Design review of the part built by this model. Coordinates are the model's own, in mm. Give positions to 0.01 mm unless a question says otherwise; leave off trailing zeros. Loops run counter-clockwise (first coordinate to the right, second up) from the corner with the lowest first, then second, coordinate; pieces in that order, holes last. Notation, with made-up numbers: (28.25, -27.75) -> (47.25, -27.75) arc R36 ccw to (47.25, 8.25) -> close; hole circle Ø11 at (-36.75, 40.5). An arc over 180 degrees is marked (long way). Answer in a Markdown table with one row per item. Add a question column.
(1) For line 1 (Y direction, x = -121.9, z = -0.15); line 2 (Y direction, x = -121.9, z = 0.45); line 3 (Y direction, x = -125, z = -2), list the stretches that pass through material, from the lowest coordinate up.
(2) Consider section B-B on z = -4.5. Write out the cut boundary in (x, y).
(3) Consider section A-A on x = 53.5. Write out the cut boundary in (y, z).
(4) For pin 1 (1.2 mm diameter, centred on y = 10.5, z = -1.5, fed in from +X); pin 2 (5 mm diameter, centred on x = -85.5, y = 19, fed in from -Z); pin 3 (2 mm diameter, centred on x = 99.5, y = 19, fed in from +Z); pin 4 (1 mm diameter, centred on x = 165.5, z = 0.5, fed in from +Y), all flat-tipped, find the tip position at first contact; note any pin that passes through.
from build123d import *

# Parameters (mm, degrees)
BOSS_EXTRUDE1_START        = 8
SKETCH2_W                  = 381
SKETCH2_H                  = 2
BOSS_EXTRUDE1_DEPTH        = 37
SKETCH3_W                  = 345
SKETCH3_H                  = 2
BOSS_EXTRUDE2_DEPTH        = 6
SKETCH4_W                  = 40.623
SKETCH4_H                  = 17.5
CUT_EXTRUDE1_DEPTH         = 3
F_6_CLEARANCE_HOLE1_D      = 3.6576
FILLET2_R                  = 5
FILLET3_R                  = 3
SKETCH8_W                  = 2
SKETCH8_H                  = 4
CUT_EXTRUDE2_DEPTH         = 196.834751768
FLATTEN_BENDS1_START       = -7
FLATTEN_BENDS1_OUTLINE_W   = 345
FLATTEN_BENDS1_OUTLINE_H   = 2
FLATTEN_BENDS1_DEPTH       = 6
FLATTEN_BENDS1_START_2     = -1
FLATTEN_BENDS1_2_OUTLINE_W = 345
FLATTEN_BENDS1_2_OUTLINE_H = 4.701769682
FLATTEN_BENDS1_2_DEPTH     = 2
PROCESS_BENDS1_START       = -172.5
PROCESS_BENDS1_DEPTH       = 345
PROCESS_BENDS1_2_DEPTH     = 345


# Read off the part's stored shape, not the designer's step: Flatten-Bends1, Process-Bends1
with BuildPart() as part:
    # Sketch2 → Boss-Extrude1 (new body)
    with BuildSketch(Plane(origin=(0, 0, 0), x_dir=(1, 0, 0), z_dir=(0, 1, 0)).offset(BOSS_EXTRUDE1_START)):
        Rectangle(SKETCH2_W, SKETCH2_H)
    extrude(amount=BOSS_EXTRUDE1_DEPTH)

    # Sketch3 → Boss-Extrude2 (add)
    with BuildSketch(Plane(origin=(0, 0, -1), x_dir=(-1, 0, 0), z_dir=(0, 0, -1))):
        with Locations((0, 9)):
            Rectangle(SKETCH3_W, SKETCH3_H)
    extrude(amount=BOSS_EXTRUDE2_DEPTH)

    # Sketch4 → Cut-Extrude1 (cut)
    with BuildSketch(Plane.XY.offset(1)):
        with Locations((170.1885, 36.25)):
            Rectangle(SKETCH4_W, SKETCH4_H)
        with Locations((-170.1885, 36.25)):
            Rectangle(SKETCH4_W, SKETCH4_H)
    extrude(amount=-CUT_EXTRUDE1_DEPTH, mode=Mode.SUBTRACT)

    # #6 Clearance Hole1 (through all)
    with Locations(Plane.XY.offset(1)):
        with Locations((-121.9, 35), (-121.9, 19), (-85.5, 35), (-85.5, 19), (99.5, 19), (99.5, 35), (135.9, 35), (135.9, 19)):
            Hole(F_6_CLEARANCE_HOLE1_D / 2)

    # Fillet2
    fillet2_edges = [part.edges().sort_by_distance(p)[0] for p in [
        (-190.5, 27.5, 0),
        (-149.877, 45, 0),
        (190.5, 27.5, 0),
        (149.877, 45, 0),
        (-190.5, 8, 0),
        (190.5, 8, 0),
    ]]
    fillet(fillet2_edges, radius=FILLET2_R)

    # Fillet3
    fillet3_edges = [part.edges().sort_by_distance(p)[0] for p in [
        (-149.877, 27.5, 0),
        (149.877, 27.5, 0),
    ]]
    fillet(fillet3_edges, radius=FILLET3_R)

    # Sketch8 → Cut-Extrude2 (cut, through all)
    with BuildSketch(Plane(origin=(0, 0, -1), x_dir=(-1, 0, 0), z_dir=(0, 0, -1))):
        with Locations((173.5, 10)):
            Rectangle(SKETCH8_W, SKETCH8_H)
        with Locations((-173.5, 10)):
            Rectangle(SKETCH8_W, SKETCH8_H)
    extrude(amount=-CUT_EXTRUDE2_DEPTH, mode=Mode.SUBTRACT)

    # Flatten-Bends1 outline → Flatten-Bends1 (cut)
    with BuildSketch(Plane.XY.offset(FLATTEN_BENDS1_START)):
        with Locations((0, 9)):
            Rectangle(FLATTEN_BENDS1_OUTLINE_W, FLATTEN_BENDS1_OUTLINE_H)
    extrude(amount=FLATTEN_BENDS1_DEPTH, mode=Mode.SUBTRACT)

    # Flatten-Bends1 2 outline → Flatten-Bends1 2 (add)
    with BuildSketch(Plane.XY.offset(FLATTEN_BENDS1_START_2)):
        with Locations((0, 5.649115159)):
            Rectangle(FLATTEN_BENDS1_2_OUTLINE_W, FLATTEN_BENDS1_2_OUTLINE_H)
    extrude(amount=FLATTEN_BENDS1_2_DEPTH)

    # Process-Bends1 outline → Process-Bends1 (cut)
    with BuildSketch(Plane.YZ.offset(PROCESS_BENDS1_START)):
        with BuildLine():
            Line((3.298230318, -1), (8.171572875, -1))
            ThreePointArc((8.171572875, -1), (9.267949192, 0.449489743), (11, 1))
            Line((11, 1), (3.298230318, 1))
            Line((3.298230318, 1), (3.298230318, -1))
        make_face()
    extrude(amount=PROCESS_BENDS1_DEPTH, mode=Mode.SUBTRACT)

    # Process-Bends1 2 outline → Process-Bends1 2 (add)
    with BuildSketch(Plane.YZ.offset(PROCESS_BENDS1_START)):
        with BuildLine():
            Line((8, -2), (8, -7))
            Line((8, -7), (10, -7))
            Line((10, -7), (10, -2))
            ThreePointArc((10, -2), (10.292893219, -1.292893219), (11, -1))
            Line((11, -1), (8.171572875, -1))
            ThreePointArc((8.171572875, -1), (8.043204321, -1.492694064), (8, -2))
        make_face()
    extrude(amount=PROCESS_BENDS1_2_DEPTH)


solid = part.part
Values follow:
| question | item | result |
|---|---|---|
| 1 | line 1 | 8.64 to 17.17, 20.83 to 33.17, 36.83 to 45 |
| 1 | line 2 | 9.27 to 17.17, 20.83 to 33.17, 36.83 to 45 |
| 1 | line 3 | 8 to 10 |
| 2 | outline | (-172.5, 8) -> (172.5, 8) -> (172.5, 10) -> (-172.5, 10) -> close |
| 3 | outline | (8, -7) -> (10, -7) -> (10, -2) arc R1 cw to (11, -1) -> (45, -1) -> (45, 1) -> (11, 1) arc R3 ccw to (8, -2) -> close |
| 4 | pin 1 | x = 190.01 |
| 4 | pin 2 | z = -1 |
| 4 | pin 3 | through |
| 4 | pin 4 | y = 27.5 |
